from build123d import *

# Parameters (mm, degrees)
SKETCH1_R                   = 25
SKETCH1_R_2                 = 15
SKETCH1_R_3                 = 10
BOSS_EXTRUDE1_DEPTH         = 80
SKETCH1_3_R                 = 15
SKETCH1_3_R_2               = 10
BOSS_EXTRUDE2_DEPTH         = 70
SKETCH1_4_R                 = 45
SKETCH1_4_R_2               = 25
BOSS_EXTRUDE3_DEPTH         = 3
M3_TAPPED_HOLE1_D           = 2.5
M3_TAPPED_HOLE1_CSINK_D     = 3.05
M3_TAPPED_HOLE1_CSINK_ANGLE = 90


with BuildPart() as part:
    # Sketch1 → Boss-Extrude1 (new body)
    # profile 1 of 2: a face of its own
    with BuildSketch(Plane(origin=(0, 0, 0), x_dir=(0, 0, -1), z_dir=(1, 0, 0))):
        Circle(SKETCH1_R)
        Circle(SKETCH1_R_2, mode=Mode.SUBTRACT)
    # profile 2 of 2: a face of its own
    with BuildSketch(Plane(origin=(0, 0, 0), x_dir=(0, 0, -1), z_dir=(1, 0, 0))):
        Circle(SKETCH1_R_2)
        Circle(SKETCH1_R_3, mode=Mode.SUBTRACT)
    extrude(amount=-BOSS_EXTRUDE1_DEPTH)



with BuildPart() as body_2:
    # Sketch1_3 → Boss-Extrude2 (new body)
    with BuildSketch(Plane(origin=(0, 0, 0), x_dir=(0, 0, -1), z_dir=(1, 0, 0))):
        Circle(SKETCH1_3_R)
        Circle(SKETCH1_3_R_2, mode=Mode.SUBTRACT)
    extrude(amount=BOSS_EXTRUDE2_DEPTH)


with BuildPart() as part_1:
    add(part.part)

    add(body_2.part)  # Boss-Extrude3 merges body 2
    # Sketch1_4 → Boss-Extrude3 (add)
    with BuildSketch(Plane(origin=(0, 0, 0), x_dir=(0, 0, -1), z_dir=(1, 0, 0))):
        Circle(SKETCH1_4_R)
        Circle(SKETCH1_4_R_2, mode=Mode.SUBTRACT)
    extrude(amount=-BOSS_EXTRUDE3_DEPTH)

    # M3 Tapped Hole1 (through all)
    with Locations(Plane.ZY.offset(3)):
        with Locations((35, 0), (0, 35), (-35, 0), (0, -35), (24.748737342, 24.748737342), (-24.748737342, 24.748737342), (-24.748737342, -24.748737342), (24.748737342, -24.748737342)):
            CounterSinkHole(M3_TAPPED_HOLE1_D / 2, M3_TAPPED_HOLE1_CSINK_D / 2, counter_sink_angle=M3_TAPPED_HOLE1_CSINK_ANGLE)


solid = part_1.part
Can you work these out from the model? Positions are in its coordinate system, mm. A direction names the side the tool comes from. Round coordinates to 2 decimals unless told otherwise and drop trailing zeros. Write each loop counter-clockwise with the first axis right and the second up, starting at its lowest first coordinate (ties: lowest second). Pieces come first, ordered by that corner, then holes. Notation, with made-up numbers: M -25.75,-19.75 L 19.25,-19.75 A19 ccw 19.25,-15.75 Z; hole C -17,19.5 d6. An arc over 180 degrees is marked long. Use a Markdown table: item, result.
Item 1: I want a section at B-B (z = 21.5). List the corners of the cut face in (x, y) for me.
Found:
| item | result |
|---|---|
| outline | M -80,-12.76 L -3,-12.76 L -3,-39.53 L 0,-39.53 L 0,39.53 L -3,39.53 L -3,12.76 L -80,12.76 Z |
Item 2: Which directions (+Z, -Z, +X, -X, +Y, -Y) give clear straight access to the entire face, cutting with the end or side of a thin tool? Please do faces 4 (the face through (-3, -19, -19)), 5 (the face through (-1.479, -39.923, -20.765)), 6 (the face through (34.51, 0.66, 14.985)).
Found:
| item | result |
|---|---|
| face 4 | -X |
| face 5 | +X, -X |
| face 6 | +X |
Item 3: We'd pull the mould along Y, two halves only. Please class faces 1 (the face through (-6.05, -9.76, 2.17)), 2 (the face through (70, -10, -3)), 3 (the face through (-40.961, 7.509, -23.846)): released by +Y, released by -Y, zero draft, split by the parting line, or undercut.
Found:
| item | result |
|---|---|
| face 1 | undercut |
| face 2 | zero draft |
| face 3 | split by the parting line |
Item 4: If I drill on line 1 along Y through (x, z) = (-39.5, 0); line 2 along X through (y, z) = (12.5, -17.5); line 3 along X through (y, z) = (-38, -24), over which ranges is the centre line in solid material (lowest first)? Write a range as [from, to].
Found:
| item | result |
|---|---|
| line 1 | y = [-25, -10], [10, 25] |
| line 2 | x = [-80, 0] |
| line 3 | x = [-3, 0] |
Item 5: I want a section at A-A (y = -6). List the corners of the cut face in (x, z) for me, and give its area (3 significant figures).
Found:
| item | result |
|---|---|
| outline | M -80,-24.27 L -3,-24.27 L -3,-44.6 L 0,-44.6 L 0,-13.75 L 70,-13.75 L 70,-8 L -80,-8 Z; M -80,8 L 70,8 L 70,13.75 L 0,13.75 L 0,44.6 L -3,44.6 L -3,24.27 L -80,24.27 Z |
| area | 3,530 mm2 |
Item 6: I want a section at C-C (x = -36.5). List the corners of the cut face in (y, z) for me, and give its area (3 significant figures).
Found:
| item | result |
|---|---|
| outline | C 0,0 d50; hole C 0,0 d20 |
| area | 1,650 mm2 |
Item 7: I want a section at D-D (x = 42). List the corners of the cut face in (y, z) for me.
Found:
| item | result |
|---|---|
| outline | C 0,0 d30; hole C 0,0 d20 |
Item 8: For pin 1 Ø16 at (y, z) = (0, 0) entering from -X; pin 2 Ø8 at (y, z) = (29, 33.5) entering from -X; pin 3 Ø1 at (x, z) = (42.5, -4.5) entering from -Y; pin 4 Ø6 at (x, y) = (-5.5, -13) entering from -Z, each with a flat end and sliding along its axis, tell me the tip position at first contact or that it passes through.
Found:
| item | result |
|---|---|
| pin 1 | passes through |
| pin 2 | stops at x = -3 |
| pin 3 | stops at y = -14.46 |
| pin 4 | stops at z = -43.55 |
